from build123d import *

# Parameters (mm, degrees)
F0_W      = 38.1
F0_H      = 38.1
F1_DEPTH  = 12.7
F2_W      = 34.925
F2_H      = 34.925
F3_DEPTH  = 9.525
F4_W      = 9.525
F4_H      = 12.7
F5_DEPTH  = 4.7625
F7_D      = 0.508
F7_DEPTH  = 14.2875
F7_TIP    = 0.1526185972
F9_D      = 0.508
F9_DEPTH  = 14.2875
F9_TIP    = 0.1526185972
F10_R     = 3.175
F15_D     = 3.175
F17_DEPTH = 0.79375
F18_R     = 0.508
F19_R     = 0.635
F20_DEPTH = 15.875
F21_R     = 0.635
F22_DEPTH = 15.875


with BuildPart() as f1:
    # F0 (on Top) → F1 (new body)
    with BuildSketch(Plane.XY):
        Rectangle(F0_W, F0_H)
    extrude(amount=F1_DEPTH)

    # F2 (on face) → F3 (cut)
    with BuildSketch(Plane.XY.offset(12.7)):
        Rectangle(F2_W, F2_H)
    extrude(amount=-F3_DEPTH, mode=Mode.SUBTRACT)

    # F4 (on face) → F5 (join)
    with BuildSketch(Plane.XY.offset(3.175)):
        Rectangle(F4_W, F4_H)
    extrude(amount=F5_DEPTH)

    # F7
    with Locations(Plane.XZ.offset(19.05)):
        with Locations((0, 6.35)):
            Hole(F7_D / 2, depth=F7_DEPTH)
            with Locations((0, 0, -(F7_DEPTH + F7_TIP / 2))):  # 118° drill point
                Cone(0, F7_D / 2, F7_TIP, mode=Mode.SUBTRACT)

    # F9
    with Locations(Plane(origin=(0, 19.05, 0), x_dir=(-1, 0, 0), z_dir=(0, 1, 0))):
        with Locations((0, 6.35)):
            Hole(F9_D / 2, depth=F9_DEPTH)
            with Locations((0, 0, -(F9_DEPTH + F9_TIP / 2))):  # 118° drill point
                Cone(0, F9_D / 2, F9_TIP, mode=Mode.SUBTRACT)

    # F10
    f10_edges = [f1.edges().sort_by_distance(p)[0] for p in [
        (-17.4625, 17.4625, 7.9375),
        (-17.4625, -17.4625, 7.9375),
        (17.4625, -17.4625, 7.9375),
        (17.4625, 17.4625, 7.9375),
    ]]
    fillet(f10_edges, radius=F10_R)

    # F13: sweep along a path in F11
    with BuildLine(Plane.XY.offset(3.175)) as f13_path:
        Line((4.7625, -7.9375), (-4.7625, -7.9375))
        ThreePointArc((-4.7625, -7.9375), (-5.8850320151, -7.4725320151), (-6.35, -6.35))
        Line((-6.35, -6.35), (-6.35, 0))
        Line((-6.35, 0), (-6.35, 6.35))
        ThreePointArc((-6.35, 6.35), (-5.8850320151, 7.4725320151), (-4.7625, 7.9375))
        Line((-4.7625, 7.9375), (4.7625, 7.9375))
        ThreePointArc((4.7625, 7.9375), (5.8850320151, 7.4725320151), (6.35, 6.35))
        Line((6.35, 6.35), (6.35, -6.35))
        ThreePointArc((6.35, -6.35), (5.8850320151, -7.4725320151), (4.7625, -7.9375))
    # F12 (on Front) → F13 (sweep, cut)
    with BuildSketch(Plane.XZ):
        with BuildLine():
            Line((-5.969, 3.175), (-6.731, 3.175))
            ThreePointArc((-6.731, 3.175), (-6.35, 2.794), (-5.969, 3.175))
        make_face()
    sweep(path=f13_path.line, mode=Mode.SUBTRACT)

    # F15 (through all)
    with Locations(Plane.XY.offset(3.175)):
        with Locations((11.8219737159, -12.2742969073), (11.8219737159, 12.2742969073), (-11.8219737159, 12.2742969073), (-11.8218979341, -12.2742284023)):
            Hole(F15_D / 2)

    # F16 (on face) → F17 (join)
    with BuildSketch(Plane.XY.offset(3.175)):
        Polygon((10.2344737159, -0.9165435523), (13.4094737159, -0.9165435523), (11.8219737159, 1.8330871047), align=None)
    extrude(amount=F17_DEPTH)

    # F18
    f18_edges = [f1.edges().sort_by_distance(p)[0] for p in [
        (11.821974, 1.833087, 3.571875),
        (13.409474, -0.916544, 3.571875),
        (10.234474, -0.916544, 3.571875),
    ]]
    fillet(f18_edges, radius=F18_R)

    # F19 (on face) → F20 (cut)
    with BuildSketch(Plane.YZ.offset(19.05)):
        with Locations((-3.175, 4.7625)):
            Circle(F19_R)
    extrude(amount=-F20_DEPTH, mode=Mode.SUBTRACT)

    # F21 (on face) → F22 (cut)
    with BuildSketch(Plane(origin=(-19.05, 0, 0), x_dir=(0, -1, 0), z_dir=(-1, 0, 0))):
        with Locations((-3.175, 4.7625)):
            Circle(F21_R)
    extrude(amount=-F22_DEPTH, mode=Mode.SUBTRACT)


solid = f1.part
The model under review builds one solid part; all positions refer to its coordinate system, in mm. A direction names the side the tool comes from. Give positions to 0.01 mm unless a question says otherwise; leave off trailing zeros. One line per question, with ' | ' between items. Start each with the question number.
Item 1: We need section B-B on x = -12.5. Give the number of separate pieces and of enclosed holes in the cut face, plus the area to 3 significant figures.
Item 2: Draft analysis for pull direction X (two halves, no side actions). For faces 1 (the cylindrical face through (-18.27, 3.31, 4.14)), 2 (the flat face through (3.175, -3, 5)), 3 (the flat face through (-8, 0, 3.175)), 4 (the flat face through (4.762, 0, 6)), state which applies: released by +X, released by -X, zero draft, split by the parting line, or undercut.
Item 3: Wall thickness on line 1 (Y direction, x = -2, z = 7.5); line 2 (X direction, y = 5.4, z = 6.35); line 3 (X direction, y = -5, z = 4.75): over which ranges is each line inside the solid? List them lowest first. Write a range as from..to.
Item 4: For pin 1 (3.5 mm diameter, centred on x = -1, y = 2, fed in from +Z); pin 2 (4 mm diameter, centred on x = -6.5, y = 8, fed in from +Z) (3 decimals), all flat-tipped, find the tip position at first contact; note any pin that passes through.
Item 5: For faces 5 (the flat face through (-0.1, 6.35, 5.5)), 6 (the cylindrical face through (10.356, -12.882, 1.565)), 7 (the cylindrical face through (3.98, -3.31, 4.14)), list the 3-axis set-ups (+Z, -Z, +X, -X, +Y, -Y) from which the entire face can be reached by the end or side of a thin tool; tool diameter is ignored.
Results found:
1) separate pieces: 3 | enclosed holes: 0 | area: 133 mm2
2) face 1: zero draft | face 2: released by +X | face 3: undercut | face 4: undercut
3) line 1: y = -19.05..-17.46, -6.35..6.35, 17.46..19.05 | line 2: x = -19.05..-17.46, -4.76..-0.25, 0.25..4.76, 17.46..19.05 | line 3: x = -19.05..-17.46, -4.76..4.76, 17.46..19.05
4) pin 1: stops at z = 7.94 | pin 2: stops at z = 3.175
5) face 5: +Z | face 6: +Z, -Z | face 7: +X
